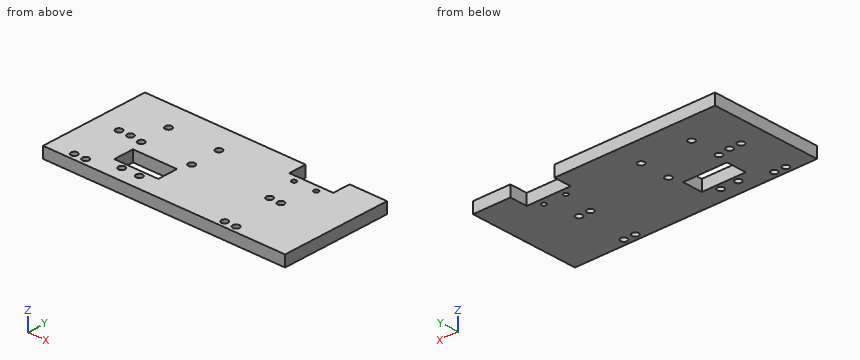
from build123d import *

# Parameters (mm, degrees)
SKETCH1_W                     = 254
SKETCH1_H                     = 63.5
BOSS_EXTRUDE1_DEPTH           = 6.35
F_6_CLEARANCE_HOLE1_D         = 3.7973
F_6_CLEARANCE_HOLE1_DEPTH     = 6.35
F_6_CLEARANCE_HOLE1_TIP       = 1.140824014
F_6_CLEARANCE_HOLE2_D         = 3.7973
F_6_CLEARANCE_HOLE2_DEPTH     = 7.62
F_6_CLEARANCE_HOLE2_TIP       = 1.140824014
SKETCH21_W                    = 12.7
SKETCH21_H                    = 11.684
CUT_EXTRUDE7_DEPTH            = 132.062523247
F_6_CLEARANCE_HOLE3_D         = 3.7973
F_6_CLEARANCE_HOLE3_DEPTH     = 7.62
F_6_CLEARANCE_HOLE3_TIP       = 1.140824014
F_6_CLEARANCE_HOLE4_D         = 3.7973
F_6_CLEARANCE_HOLE4_DEPTH     = 7.62
F_6_CLEARANCE_HOLE4_TIP       = 1.140824014
SKETCH27_W                    = 114.3
SKETCH27_H                    = 63.5
CUT_EXTRUDE9_DEPTH            = 132.062523247
SKETCH28_W                    = 25.4
SKETCH28_H                    = 10.16
CUT_EXTRUDE10_DEPTH           = 33.02
TAP_DRILL_FOR_6_32_TAP1_D     = 2.7051
TAP_DRILL_FOR_6_32_TAP1_DEPTH = 10.16
TAP_DRILL_FOR_6_32_TAP1_TIP   = 0.81269403
F_6_CLEARANCE_HOLE5_D         = 3.7973
F_6_CLEARANCE_HOLE5_DEPTH     = 10.16
F_6_CLEARANCE_HOLE5_TIP       = 1.140824014


with BuildPart() as part:
    # Sketch1 → Boss-Extrude1 (new body)
    with BuildSketch(Plane.XY):
        Rectangle(SKETCH1_W, SKETCH1_H)
    extrude(amount=BOSS_EXTRUDE1_DEPTH)

    # #6 Clearance Hole1
    with Locations(Plane.XY.offset(6.35)):
        with Locations((-105.918, 0), (-112.522, -27.94), (-112.522, 0), (-105.918, -27.94)):
            Hole(F_6_CLEARANCE_HOLE1_D / 2, depth=F_6_CLEARANCE_HOLE1_DEPTH)
            with Locations((0, 0, -(F_6_CLEARANCE_HOLE1_DEPTH + F_6_CLEARANCE_HOLE1_TIP / 2))):  # 118° drill point
                Cone(0, F_6_CLEARANCE_HOLE1_D / 2, F_6_CLEARANCE_HOLE1_TIP, mode=Mode.SUBTRACT)

    # #6 Clearance Hole2
    with Locations(Plane(origin=(0, 0, 0), x_dir=(-1, 0, 0), z_dir=(0, 0, -1))):
        with Locations((98.806, -1.016), (69.723, -1.016)):
            Hole(F_6_CLEARANCE_HOLE2_D / 2, depth=F_6_CLEARANCE_HOLE2_DEPTH)
            with Locations((0, 0, -(F_6_CLEARANCE_HOLE2_DEPTH + F_6_CLEARANCE_HOLE2_TIP / 2))):  # 118° drill point
                Cone(0, F_6_CLEARANCE_HOLE2_D / 2, F_6_CLEARANCE_HOLE2_TIP, mode=Mode.SUBTRACT)

    # Sketch21 → Cut-Extrude7 (cut, through all)
    with BuildSketch(Plane(origin=(0, 0, 0), x_dir=(-1, 0, 0), z_dir=(0, 0, -1))):
        with Locations((77.9145, -13.97)):
            Rectangle(SKETCH21_W, SKETCH21_H)
        with Locations((90.6145, -13.97)):
            Rectangle(SKETCH21_W, SKETCH21_H)
    extrude(amount=-CUT_EXTRUDE7_DEPTH, mode=Mode.SUBTRACT)

    # #6 Clearance Hole3
    with Locations(Plane(origin=(0, 0, 0), x_dir=(-1, 0, 0), z_dir=(0, 0, -1))):
        with Locations((69.723, 16.002), (98.806, 16.002)):
            Hole(F_6_CLEARANCE_HOLE3_D / 2, depth=F_6_CLEARANCE_HOLE3_DEPTH)
            with Locations((0, 0, -(F_6_CLEARANCE_HOLE3_DEPTH + F_6_CLEARANCE_HOLE3_TIP / 2))):  # 118° drill point
                Cone(0, F_6_CLEARANCE_HOLE3_D / 2, F_6_CLEARANCE_HOLE3_TIP, mode=Mode.SUBTRACT)

    # #6 Clearance Hole4
    with Locations(Plane(origin=(0, 0, 0), x_dir=(-1, 0, 0), z_dir=(0, 0, -1))):
        with Locations((79.1845, -23.35276), (89.3445, -23.35276)):
            Hole(F_6_CLEARANCE_HOLE4_D / 2, depth=F_6_CLEARANCE_HOLE4_DEPTH)
            with Locations((0, 0, -(F_6_CLEARANCE_HOLE4_DEPTH + F_6_CLEARANCE_HOLE4_TIP / 2))):  # 118° drill point
                Cone(0, F_6_CLEARANCE_HOLE4_D / 2, F_6_CLEARANCE_HOLE4_TIP, mode=Mode.SUBTRACT)

    # Sketch27 → Cut-Extrude9 (cut, through all)
    with BuildSketch(Plane.XY.offset(6.35)):
        with Locations((69.85, 0)):
            Rectangle(SKETCH27_W, SKETCH27_H)
    extrude(amount=-CUT_EXTRUDE9_DEPTH, mode=Mode.SUBTRACT)

    # Sketch28 → Cut-Extrude10 (cut)
    with BuildSketch(Plane.XY.offset(6.35)):
        with Locations((-21.59, 26.67)):
            Rectangle(SKETCH28_W, SKETCH28_H)
    extrude(amount=-CUT_EXTRUDE10_DEPTH, mode=Mode.SUBTRACT)

    # Tap Drill for #6-32 Tap1
    with Locations(Plane.XY.offset(6.35)):
        with Locations((-27.94, 17.78), (-15.24, 17.78)):
            Hole(TAP_DRILL_FOR_6_32_TAP1_D / 2, depth=TAP_DRILL_FOR_6_32_TAP1_DEPTH)
            with Locations((0, 0, -(TAP_DRILL_FOR_6_32_TAP1_DEPTH + TAP_DRILL_FOR_6_32_TAP1_TIP / 2))):  # 118° drill point
                Cone(0, TAP_DRILL_FOR_6_32_TAP1_D / 2, TAP_DRILL_FOR_6_32_TAP1_TIP, mode=Mode.SUBTRACT)

    # #6 Clearance Hole5
    with Locations(Plane.XY.offset(6.35)):
        with Locations((-25.668797482, 0), (-19.064797482, 0), (-25.668797482, -27.94), (-19.064797482, -27.94)):
            Hole(F_6_CLEARANCE_HOLE5_D / 2, depth=F_6_CLEARANCE_HOLE5_DEPTH)
            with Locations((0, 0, -(F_6_CLEARANCE_HOLE5_DEPTH + F_6_CLEARANCE_HOLE5_TIP / 2))):  # 118° drill point
                Cone(0, F_6_CLEARANCE_HOLE5_D / 2, F_6_CLEARANCE_HOLE5_TIP, mode=Mode.SUBTRACT)


solid = part.part
Geometry: final body of the model. Coordinates: model frame, mm. Give positions to 0.01 mm unless a question says otherwise; leave off trailing zeros. Loops run counter-clockwise (first coordinate to the right, second up) from the corner with the lowest first, then second, coordinate; pieces in that order, holes last. Notation, with made-up numbers: (-38.75, 44.25) - (20.25, 44.25) arc R11 ccw to (20.25, 65.25) - close; hole circle Ø7 at (-8, 61). An arc over 180 degrees is marked (long way). One line per question, with ' | ' between items. Start each with the question number.
(1) Ray query, line 1 (Y direction, x = -106, z = 1); line 2 (X direction, y = -23.5, z = 4); line 3 (Y direction, x = -107, z = 5). Return the intervals inside material, ascending. Write a range as from..to.
(2) Section query B-B on y = -15.5. Return loops of the section in (x, z), then the cut area to 3 significant figures.
(3) Section query A-A on x = -15.24. Return loops of the section in (y, z).
(4) Section query C-C on z = 4. Count the separate pieces of the cut face and the enclosed holes in it, then the cut area to 3 significant figures.
(5) Contact query for flat-ended pins moving along their axis: pin 1 (3 mm diameter, centred on x = -27, z = 3.5, fed in from +Y); pin 2 (2.5 mm diameter, centred on x = -25.67, y = 0, fed in from -Z). Output: stop coordinate, or through.
The answers:
1) line 1: -31.75..-29.84, -26.04..-1.9, 1.9..31.75 | line 2: -127..-91.24, -87.45..-81.08, -77.29..12.7 | line 3: -31.75..-29.5, -26.38..-1.56, 1.56..31.75
2) outline: (-127, 0) - (-96.96, 0) - (-96.96, 6.35) - (-127, 6.35) - close; (-71.56, 0) - (12.7, 0) - (12.7, 6.35) - (-71.56, 6.35) - close | area: 726 mm2
3) outline: (-31.75, 0) - (16.43, 0) - (16.43, 6.35) - (-31.75, 6.35) - close; (19.13, 0) - (21.59, 0) - (21.59, 6.35) - (19.13, 6.35) - close
4) separate pieces: 1 | enclosed holes: 17 | area: 8,150 mm2
5) pin 1: y = 21.59 | pin 2: through
